Model file for the job. Use its own axes, mm. Face numbers are marked on the shaded views. Coordinates: 2 decimals unless noted, no trailing zeros. Write each loop counter-clockwise with the first axis right and the second up, starting at its lowest first coordinate (ties: lowest second). Pieces come first, ordered by that corner, then holes. Notation, with made-up numbers: M 45.5,79 L 51.5,79 A11 cw 51.5,92 Z; hole C -39.75,86 d9. An arc over 180 degrees is marked long. Put each result on its own line as item: value. Start each with the question number.
Q1. Cut at A-A (y = -85.5). Give the number of separate pieces and of enclosed holes in the cut face, then the cut area to 3 significant figures.
Q2. Pull direction X, two halves, no side cores. Call the marked faces 1, 2 and 3: pulls with the +X half, pulls with the -X half, needs draft (parallel to the pull), parting line crosses it, or undercut.
Q3. Cut at B-B (x = 266.5). Write the cut outline in (y, z), then the cut area to 3 significant figures.
Q4. Drill centre lines: line 1 along X through (y, z) = (-43, 188); line 2 along X through (y, z) = (-4, 188); line 3 along Y through (x, z) = (878, 314.5). Where is each one in solid material? Low to high.
Q5. Drop flat-ended pins along their axis: pin 1 (1 mm diameter, centred on x = 121, z = 248.5, fed in from -Y); pin 2 (19.5 mm diameter, centred on x = 298.89, z = 188.5, fed in from -Y). Give the stop position or say it passes through.
Q6. Cut at C-C (z = 91). Write the cut outline in (x, y), then the cut area to 3 significant figures.
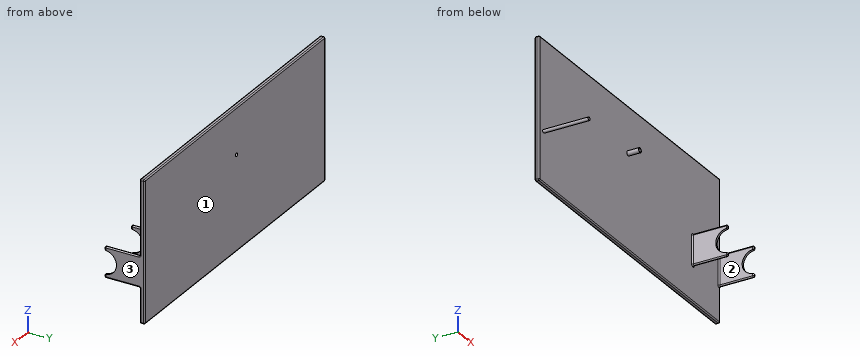
```python
from build123d import *

# Parameters (mm, degrees)
F0_W      = 1300
F0_H      = 214.1299426556
F0_H_2    = 385.8700573444
F1_DEPTH  = 20
F2_W      = 5
F2_H      = 130
F3_DEPTH  = 150
F4_R      = 50
F5_DEPTH  = 2015
F6_R      = 4.99999
F7_R      = 7.5
F8_DEPTH  = 20.001
F7_R_2    = 10
F9_DEPTH  = 50
F10_R     = 7
F11_DEPTH = 194


# Not quite as in the source:
# - a fillet or chamfer is up to 0.001 mm smaller than in the source, because OpenCascade refuses the exact size


with BuildPart() as f1:
    # F0 (on Front) → F1 (new body)
    with BuildSketch(Plane.XZ):
        with Locations((309.8854213953, -107.0649713278)):
            Rectangle(F0_W, F0_H)
        with Locations((309.8854213953, 192.9350286722)):
            Rectangle(F0_W, F0_H_2)
    extrude(amount=F1_DEPTH)

    # F2 (on face) → F3 (join)
    with BuildSketch(Plane.XZ.offset(20)):
        Polygon((949.8854213953, 65), (949.8854213953, 0), (949.8854213953, -65), (954.8854213953, -65), (954.8854213953, 65), align=None)
        with Locations((762.3854213953, 0)):
            Rectangle(F2_W, F2_H)
        Polygon((769.8854213953, 65), (764.8854213953, 65), (764.8854213953, -65), (769.8854213953, -65), (769.8854213953, 0), align=None)
        with Locations((957.3854213953, 0)):
            Rectangle(F2_W, F2_H)
    extrude(amount=F3_DEPTH)

    # F4 (on face) → F5 (cut)
    with BuildSketch(Plane.YZ.offset(959.8854213953)):
        with Locations((-170, 0)):
            Circle(F4_R)
    extrude(amount=-F5_DEPTH, mode=Mode.SUBTRACT)

    # F6 (radius 5 in the source; OpenCascade refuses exactly that, so slightly less here)
    f6_edges = [f1.edges().sort_by_distance(p)[0] for p in [
        (764.885421, -170, -50),
        (769.885421, -170, -57.5),
        (764.885421, -170, -65),
        (759.885421, -170, -57.5),
        (764.885421, -170, 65),
        (769.885421, -170, 57.5),
        (764.885421, -170, 50),
        (759.885421, -170, 57.5),
        (759.885421, -95, -65),
        (769.885421, -95, -65),
        (764.885421, -20, -65),
        (769.885421, -95, 65),
        (759.885421, -95, 65),
        (764.885421, -20, 65),
        (954.885421, -170, 65),
        (959.885421, -170, 57.5),
        (954.885421, -170, 50),
        (949.885421, -170, 57.5),
        (954.885421, -170, -50),
        (959.885421, -170, -57.5),
        (954.885421, -170, -65),
        (949.885421, -170, -57.5),
        (949.885421, -95, -65),
        (959.885421, -95, -65),
        (954.885421, -20, -65),
        (959.885421, -95, 65),
        (949.885421, -95, 65),
        (954.885421, -20, 65),
        (309.885421, 0, 385.870057),
        (959.885421, -10, 385.870057),
        (-340.114579, -10, 385.870057),
        (309.885421, -20, 385.870057),
        (-340.114579, -10, -214.129943),
        (959.885421, -10, -214.129943),
        (309.885421, 0, -214.129943),
        (309.885421, -20, -214.129943),
        (959.885421, 0, 85.870057),
        (-340.114579, 0, 85.870057),
        (-340.114579, -20, 85.870057),
        (959.885421, -20, 225.435029),
        (949.885421, -20, 0),
        (959.885421, -20, -139.564971),
        (759.885421, -20, 0),
        (769.885421, -20, 0),
    ]]
    fillet(f6_edges, radius=F6_R)

    # F7 (on face) → F8 (cut, through all)
    with BuildSketch(Plane.XZ.offset(20)):
        with Locations((298.8854213953, 188.5)):
            Circle(F7_R)
    extrude(amount=-F8_DEPTH, mode=Mode.SUBTRACT)

    # F7 (on face) → F9 (join)
    with BuildSketch(Plane.XZ.offset(20)):
        with Locations((298.8854213953, 188.5)):
            Circle(F7_R_2)
        with Locations((298.8854213953, 188.5)):
            Circle(F7_R, mode=Mode.SUBTRACT)
    extrude(amount=F9_DEPTH)

    # F10 (on face) → F11 (join)
    with BuildSketch(Plane.XZ.offset(20)):
        with Locations((-310.1145786047, 0)):
            Circle(F10_R)
    extrude(amount=F11_DEPTH)


solid = f1.part
```
Computed values:
1. separate pieces: 3
1. enclosed holes: 0
1. area: 2,710 mm2
2. face 1: needs draft
2. face 2: undercut
2. face 3: pulls with the +X half
3. outline: M -20,-209.13 A5 ccw -15,-214.13 L -5,-214.13 A5 ccw 0,-209.13 L 0,380.87 A5 ccw -5,385.87 L -15,385.87 A5 ccw -20,380.87 Z
3. area: 12,000 mm2
4. line 1: 288.9 to 291.4, 306.37 to 308.87
4. line 2: -340.01 to 291.4, 306.37 to 959.78
4. line 3: -20 to 0
5. pin 1: y = -20
5. pin 2: y = -70
6. outline: M -340.11,-15 A5 ccw -335.11,-20 L 954.89,-20 A5 ccw 959.89,-15 L 959.89,-5 A5 ccw 954.89,0 L -335.11,0 A5 ccw -340.11,-5 Z
6. area: 26,000 mm2
